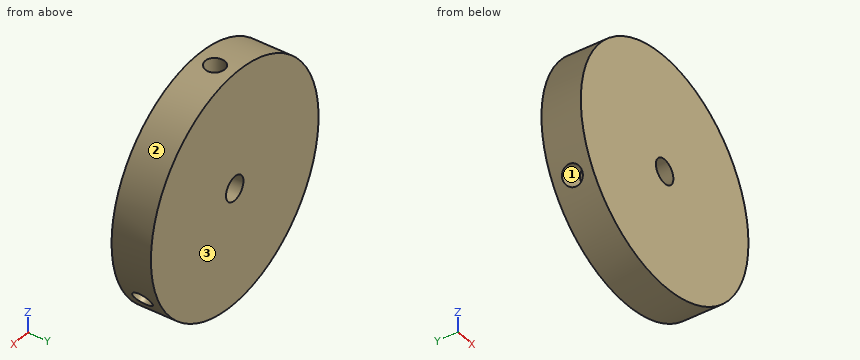
```python
from build123d import *

# Parameters (mm, degrees)
SKETCH1_R           = 38.1
BOSS_EXTRUDE1_DEPTH = 12.7
SKETCH2_R           = 3.175
CUT_EXTRUDE1_DEPTH  = 9.525
CIRPATTERN1_COUNT   = 3
SKETCH3_R           = 3.9624
CUT_EXTRUDE2_DEPTH  = 12.7


with BuildPart() as part:
    # Sketch1 → Boss-Extrude1 (new body)
    with BuildSketch(Plane(origin=(0, 0, 0), x_dir=(1, 0, 0), z_dir=(0, 1, 0))):
        Circle(SKETCH1_R)
    extrude(amount=BOSS_EXTRUDE1_DEPTH)

    # Sketch2 → Cut-Extrude1 (cut)
    with BuildSketch(Plane.XY.offset(38.1)):
        with Locations((0, 6.35)):
            Circle(SKETCH2_R)
    cut_extrude1 = extrude(amount=-CUT_EXTRUDE1_DEPTH, mode=Mode.SUBTRACT)

    # CirPattern1: Cut-Extrude1 ×3 about axis
    cirpattern1_axis = Axis((0, 0, 0), (0, 1, 0))
    for i in range(1, CIRPATTERN1_COUNT):
        add(cut_extrude1.rotate(cirpattern1_axis, i * 360 / CIRPATTERN1_COUNT), mode=Mode.SUBTRACT)

    # Sketch3 → Cut-Extrude2 (cut)
    with BuildSketch(Plane(origin=(0, 12.7, 0), x_dir=(1, 0, 0), z_dir=(0, 1, 0))):
        Circle(SKETCH3_R)
    extrude(amount=-CUT_EXTRUDE2_DEPTH, mode=Mode.SUBTRACT)


solid = part.part
```
Model file for the job. Use its own axes, mm. Face numbers are marked on the shaded views. Round coordinates to 2 decimals unless told otherwise and drop trailing zeros. Order: outer loops, then holes, each group sorted by start corner. A loop starts at its lowest first (then second) coordinate and runs counter-clockwise, first axis right, second up. Notation, with made-up numbers: (-22.5, 20) -> (1.5, 20) arc R20 cw to (1.5, 40) -> close; hole circle Ø1 at (38.25, 43.5). An arc over 180 degrees is marked (long way). Use one line per item in the form item = value.
Item 1: Cut at B-B, the plane z = 0. Write the cut outline in (x, y), and give its area (3 significant figures).
Returned:
outline = (-38.1, 0) -> (-3.96, 0) -> (-3.96, 12.7) -> (-38.1, 12.7) -> close; (3.96, 0) -> (38.1, 0) -> (38.1, 12.7) -> (3.96, 12.7) -> close
area = 867 mm^2
Item 2: Cut at D-D, the plane z = 32.5. Write the cut outline in (x, y) (3 decimals), and give its area (3 significant figures).
Returned:
outline = (-19.884, 0) -> (19.884, 0) -> (19.884, 12.7) -> (-19.884, 12.7) -> close; hole circle Ø6.35 at (0, 6.35)
area = 473 mm^2
Item 3: Cut at A-A, the plane x = 0. Write the cut outline in (y, z) (3 decimals), and give its area (3 significant figures).
Returned:
outline = (0, -38.1) -> (12.7, -38.1) -> (12.7, -3.962) -> (0, -3.962) -> close; (0, 3.962) -> (12.7, 3.962) -> (12.7, 38.1) -> (9.525, 38.1) -> (9.525, 28.575) -> (3.175, 28.575) -> (3.175, 38.1) -> (0, 38.1) -> close
area = 807 mm^2
Item 4: Drill centre lines: line 1 (Z direction, x = 0, y = 6) (3 decimals); line 2 (X direction, y = 3, z = 0); line 3 (Y direction, x = 0, z = 35) (3 decimals). Where is each one in solid material? Low to high.
Returned:
line_1 = -38.1 to -3.962, 3.962 to 28.575
line_2 = -38.1 to -3.96, 3.96 to 38.1
line_3 = 0 to 3.175, 9.525 to 12.7
Item 5: Pull direction Z, two halves, no side cores. Call the marked faces 1, 2 and 3: released by +Z, released by -Z, zero draft, split by the parting line, or undercut.
Returned:
face_1 = undercut
face_2 = split by the parting line
face_3 = zero draft
Item 6: Flat gauge pins, fed straight in: pin 1 Ø6 at (y, z) = (7.5, -7.5) entering from +X; pin 2 Ø1 at (x, y) = (-11.5, 1.5) entering from +Z; pin 3 Ø5 at (x, y) = (0, 6.35) entering from -Z. Where does each tip first touch, or does it go through?
Returned:
pin_1 = 37.83
pin_2 = 36.48
pin_3 = -38.1
Item 7: Cut at C-C, the plane y = 6.35. Write the cut outline in (x, z) (3 decimals), and give its area (3 significant figures).
Returned:
outline = (-34.468, -16.234) -> (-26.334, -11.538) -> (-23.159, -17.037) -> (-31.293, -21.733) arc R38.1 ccw to (31.293, -21.733) -> (23.159, -17.037) -> (26.334, -11.538) -> (34.468, -16.234) arc R38.1 ccw to (3.175, 37.967) -> (3.175, 28.575) -> (-3.175, 28.575) -> (-3.175, 37.967) arc R38.1 ccw to start; hole circle Ø7.925 at (0, 0)
area = 4,330 mm^2
